Verification items for this drawing (mm, ordinates from the low corner). Round coordinates to 2 decimals unless told otherwise and drop trailing zeros. Order: outer loops, then holes, each group sorted by start corner. A loop starts at its lowest first (then second) coordinate and runs counter-clockwise, first axis right, second up. Notation, with made-up numbers: (-24.75, -11.5) -> (34.25, -11.5) arc R14 cw to (34.25, 13.5) -> close; hole circle Ø8 at (19.5, -2). An arc over 180 degrees is marked (long way). Put each result on its own line as item: value.
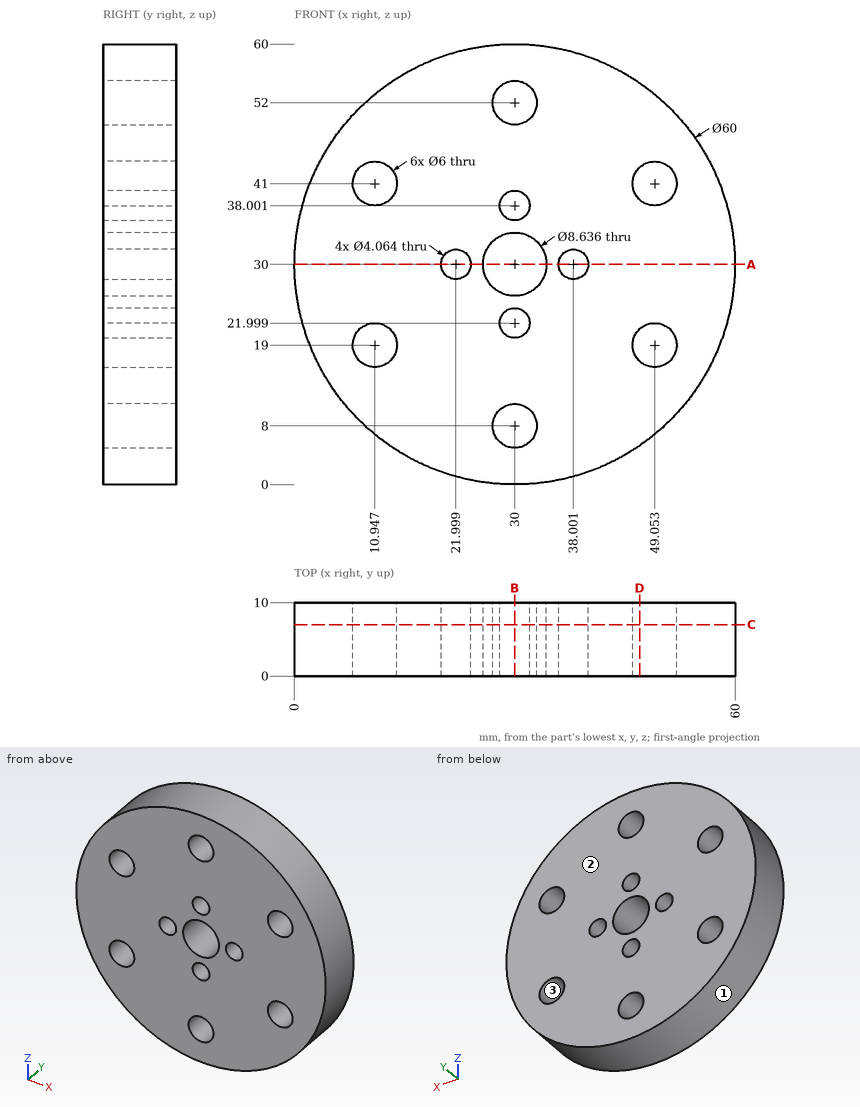
Item 1: Gauge pin test, flat ends, axial feed: pin 1 Ø3.5 at (x, z) = (38.001, 30) entering from -Y; pin 2 Ø1 at (y, z) = (2.5, 13) entering from -X (1 decimal); pin 3 Ø4 at (x, y) = (44, 8) entering from -Z (1 decimal); pin 4 Ø2 at (y, z) = (9, 9.5) entering from -X. Record the tip position at first contact, or that the pin passes through.
Check sheet entries:
pin 1: passes through
pin 2: stops at x = 4.9
pin 3: stops at z = 2.5
pin 4: stops at x = 7.2
Item 2: Section check C-C on y = 7. State how many separate pieces and enclosed holes the cut face has, then the cut area to 3 significant figures.
Check sheet entries:
separate pieces: 1
enclosed holes: 11
area: 2,550 mm^2
Item 3: Section check D-D on x = 47. Record the boundary of the cut face in (y, z).
Check sheet entries:
outline: (0, 5.28) -> (10, 5.28) -> (10, 16.81) -> (0, 16.81) -> close; (0, 21.19) -> (10, 21.19) -> (10, 38.81) -> (0, 38.81) -> close; (0, 43.19) -> (10, 43.19) -> (10, 54.72) -> (0, 54.72) -> close
Item 4: Release check for a two-part mould opening along Z. For the marked faces 1, 2 and 3 record: +Z half, -Z half, draft (parallel to the pull), parting line (faces both ways), or undercut.
Check sheet entries:
face 1: parting line
face 2: draft
face 3: undercut
Item 5: Section check B-B on x = 30. Record the boundary of the cut face in (y, z).
Check sheet entries:
outline: (0, 0) -> (10, 0) -> (10, 5) -> (0, 5) -> close; (0, 11) -> (10, 11) -> (10, 19.97) -> (0, 19.97) -> close; (0, 24.03) -> (10, 24.03) -> (10, 25.68) -> (0, 25.68) -> close; (0, 34.32) -> (10, 34.32) -> (10, 35.97) -> (0, 35.97) -> close; (0, 40.03) -> (10, 40.03) -> (10, 49) -> (0, 49) -> close; (0, 55) -> (10, 55) -> (10, 60) -> (0, 60) -> close
Item 6: Material ranges on L1, parallel to X at y = 3.75, z = 30; L2, parallel to Z at x = 9, y = 9.5 (1 decimal); L3, parallel to X at y = 3, z = 18.5 (1 decimal), recorded low to high. Write a range as [from, to].
Check sheet entries:
L1: x = [0, 19.97], [24.03, 25.68], [34.32, 35.97], [40.03, 60]
L2: z = [8.6, 16.7], [21.3, 38.7], [43.3, 51.4]
L3: x = [2.3, 8], [13.9, 46.1], [52, 57.7]
Item 7: Section check A-A on z = 30. Record the boundary of the cut face in (x, y).
Check sheet entries:
outline: (0, 0) -> (19.97, 0) -> (19.97, 10) -> (0, 10) -> close; (24.03, 0) -> (25.68, 0) -> (25.68, 10) -> (24.03, 10) -> close; (34.32, 0) -> (35.97, 0) -> (35.97, 10) -> (34.32, 10) -> close; (40.03, 0) -> (60, 0) -> (60, 10) -> (40.03, 10) -> close
